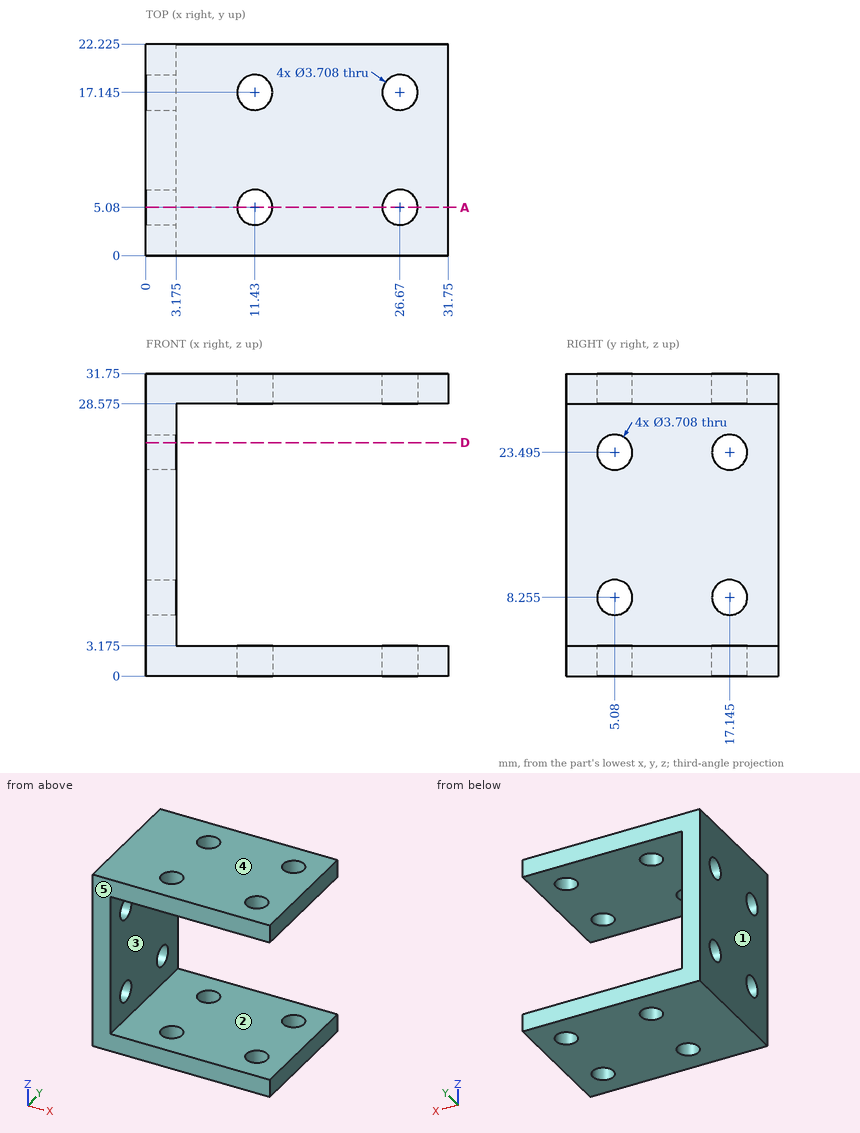
Geometry check sheet. Reference: drawing and pictorial views, mm from the part's lowest x, y, z. A direction names the side the tool comes from. Coordinates: 2 decimals unless noted, no trailing zeros. Write each loop counter-clockwise with the first axis right and the second up, starting at its lowest first coordinate (ties: lowest second). Pieces come first, ordered by that corner, then holes.
Item 1: Cross-section at D-D on z = 24.5. Record the boundary of the cut face in (x, y) (1 decimal).
Numbers:
outline: (0, 0) - (3.2, 0) - (3.2, 3.5) - (0, 3.5) - close; (0, 6.6) - (3.2, 6.6) - (3.2, 15.6) - (0, 15.6) - close; (0, 18.7) - (3.2, 18.7) - (3.2, 22.2) - (0, 22.2) - close
Item 2: Mould release check, pull along Z, two halves, no side actions. Record for the marked faces 3, 4 and 5: released by +Z, released by -Z, zero draft, split by the parting line, or undercut.
Numbers:
face 3: undercut
face 4: released by +Z
face 5: zero draft
Item 3: Depth check by flat-ended pin: pin 1 Ø1.5 at (y, z) = (10.5, 22) entering from +X (3 decimals). Enter the tip coordinate at first touch or a pass-through.
Numbers:
pin 1: stops at x = 3.175
Item 4: Scan lines: probe 1 along Y at (x, z) = (26.67, 29.6) (1 decimal); probe 2 along X at (y, z) = (19, 3.5) (1 decimal); probe 3 along Y at (x, z) = (2.5, 9) (1 decimal). Record each from-to range of solid material in increasing order.
Numbers:
probe 1: y = 0 to 3.2, 6.9 to 15.3, 19 to 22.2
probe 2: x = 0 to 3.2
probe 3: y = 0 to 3.4, 6.8 to 15.4, 18.8 to 22.2
Item 5: Access from +Z, -Z, +X, -X, +Y, -Y to the whole of each face (thin tool, end or side, straight path). Record for the marked faces 1 and 2.
Numbers:
face 1: +Z, -Z, -X, +Y, -Y
face 2: +X, +Y, -Y
Item 6: Cross-section at A-A on y = 5.08. Count the separate pieces of the cut face and the enclosed holes in it.
Numbers:
separate pieces: 7
enclosed holes: 0
